Part print with two shaded views. Sizes in mm from the minimum x, y, z corner. A direction names the side the tool comes from. Give positions to 0.01 mm unless a question says otherwise; leave off trailing zeros. Order: outer loops, then holes, each group sorted by start corner. A loop starts at its lowest first (then second) coordinate and runs counter-clockwise, first axis right, second up. Notation, with made-up numbers: (33, 83.5) - (73, 83.5) arc R16 cw to (73, 110.5) - close; hole circle Ø2 at (57, 86.25). An arc over 180 degrees is marked (long way). Return JSON: item names as keys, results as strings. Group by question number.
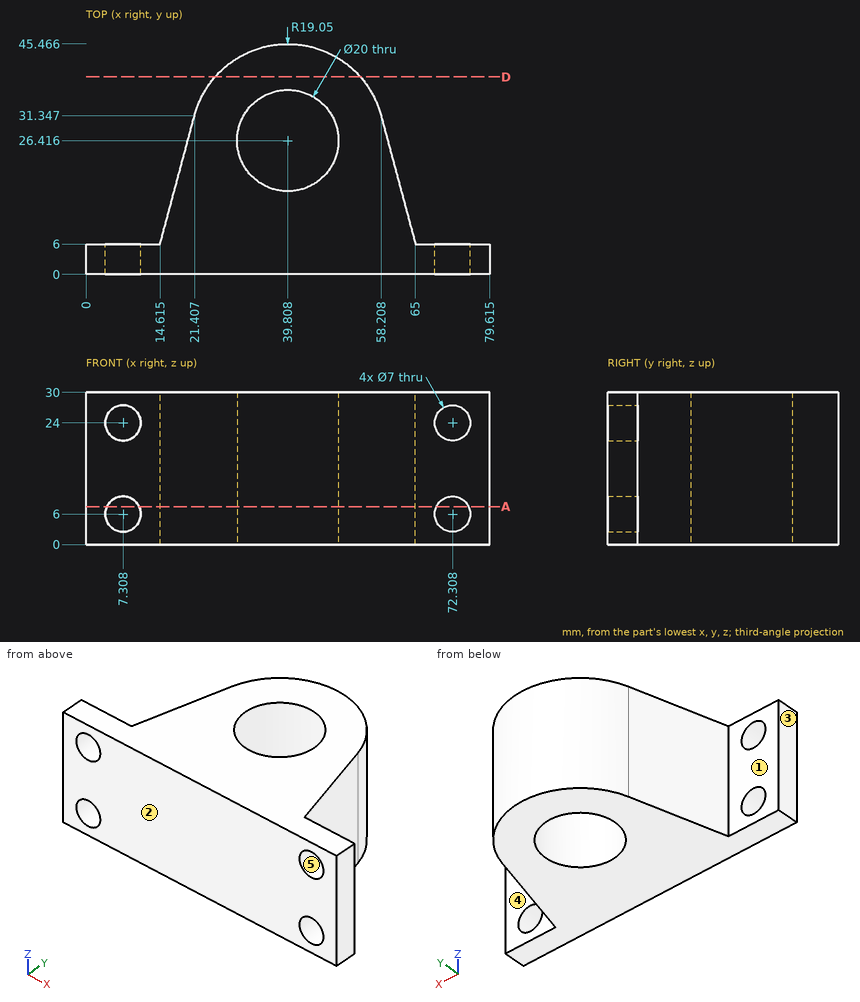
(1) Slice it at A-A (z = 7.5). State how many separate pieces and enclosed holes the cut face has, and give its area (3 significant figures).
(2) 3-axis set-ups, long thin cutter, end or side, ignore diameter. For the marked faces 1 and 2: which of +Z, -Z, +X, -X, +Y, -Y reach the whole face in a straight line?
(3) Drill centre lines: L1, parallel to X at y = 3.7, z = 6 (1 decimal); L2, parallel to Y at x = 66.5, z = 8.25; L3, parallel to Y at x = 44, z = 25.75 (1 decimal). Where is each one in solid material? Low to high.
(4) Slice it at D-D (y = 39). Give the cut face in (x, z) (1 decimal), and give its area (3 significant figures).
(5) Pull direction X, two halves, no side cores. Call the marked faces 3, 4 and 5: released by +X, released by -X, zero draft, split by the parting line, or undercut.
(6) Drop flat-ended pins along their axis: pin 1 Ø4.5 at (x, z) = (10, 17) entering from +Y; pin 2 Ø12 at (x, z) = (56, 22) entering from +Y; pin 3 Ø6 at (x, z) = (43, 11) entering from +Y (1 decimal); pin 4 Ø4 at (x, z) = (72.31, 6) entering from +Y. Give the stop position or say it passes through.
Result set:
{
 "1": {"separate pieces": "3", "enclosed holes": "1", "area": "1,580 mm²"},
 "2": {"face 1": "+Z, -Z, -X, +Y", "face 2": "+Z, -Z, +X, -X, -Y"},
 "3": {"L1": "x = 0 to 3.8, 10.8 to 68.8, 75.8 to 79.6", "L2": "y = 0 to 6", "L3": "y = 0 to 17.3, 35.5 to 45"},
 "4": {"outline": "(25.5, 0) - (54.1, 0) - (54.1, 30) - (25.5, 30) - close", "area": "858 mm²"},
 "5": {"face 3": "released by -X", "face 4": "zero draft", "face 5": "undercut"},
 "6": {"pin 1": "stops at y = 6", "pin 2": "stops at y = 42.51", "pin 3": "stops at y = 45.5", "pin 4": "passes through"}
}
